Here's how the part is built. I have some questions about the finished solid (model axes, mm). Coordinates: 2 decimals unless noted, no trailing zeros. Write each loop counter-clockwise with the first axis right and the second up, starting at its lowest first coordinate (ties: lowest second). Pieces come first, ordered by that corner, then holes. Notation, with made-up numbers: (-18, 73.25) -> (1, 73.25) arc R19 cw to (1, 89.25) -> close; hole circle Ø8 at (-25, -38.75). An arc over 180 degrees is marked (long way). Use a Markdown table: item, result. Add a question column.
Item 1: If we mould it in two halves opening along Y, with no side actions, what happens to faces 1 (the cylindrical face through (-0.867, 3.905, 4.933)), 2 (the flat face through (2, 1, 10)), 3 (the cylindrical face through (1.438, -0.748, 4.933))? For each: pulls with the +Y half, pulls with the -Y half, needs draft (parallel to the pull), parting line crosses it, or undercut.
Item 2: If I drill on line 1 along Y through (x, z) = (0, 4.75); line 2 along X through (y, z) = (1, 4.5); line 3 along Y through (x, z) = (2.5, 3), over which ranges is the centre line in solid material (lowest first)? Write a range as from..to.
Item 3: Will these pins go through, and if not, where does the flat tip stop? pin 1 Ø1 at (y, z) = (1, 8.5) entering from -X; pin 2 Ø3.5 at (x, y) = (0, 0) entering from +Z.
Item 4: Imagine slicing it at A-A, the plane x = 0. Write out the boundary of the cut face in (y, z).
Item 5: Imagine slicing it at C-C, the plane z = 0.75. Write out the boundary of the cut face in (x, y), and give its area (3 significant figures).
Autodesk Inventor part; units mm, degrees
ref_plane "YZ Plane" through (0, 0, 0) normal (1, 0, 0) x (0, 1, 0)
ref_plane "XZ Plane" through (0, 0, 0) normal (0, 1, 0) x (-1, 0, 0)
ref_plane "XY Plane" through (0, 0, 0) normal (0, 0, 1) x (1, 0, 0)
sketch "スケッチ1" plane through (0, 0, 0) normal (0, 0, 1) x (1, 0, 0)
  circle A0 centre (0, 0) radius 4
  dimension "d13" = 8
extrude "押し出し1" add sketch "スケッチ1" along normal blind 10
sketch "スケッチ2" plane through (0, 0, 10) normal (0, 0, 1) x (1, 0, 0)
  point P0 (0, 0)
  point P1 (0, 0)
hole "穴1" at (0, 0, 10) direction (0, 0, -1) diameter 3.242 end through all
chamfer "面取り1" distance 0.2 angle 45 4 edges at (0, 1.621, 10) (0, 1.621, 0) (-4, 0, 10) (-4, 0, 0)
properties part number "ARF-410E" material "鋼、炭素鋼"
Ans:
| question | item | result |
|---|---|---|
| 1 | face 1 | parting line crosses it |
| 1 | face 2 | needs draft |
| 1 | face 3 | undercut |
| 2 | line 1 | y = -4..-1.62, 1.62..4 |
| 2 | line 2 | x = -3.87..-1.28, 1.28..3.87 |
| 2 | line 3 | y = -3.12..3.12 |
| 3 | pin 1 | stops at x = -3.97 |
| 3 | pin 2 | stops at z = 9.93 |
| 4 | outline | (-4, 0.2) -> (-3.8, 0) -> (-1.82, 0) -> (-1.62, 0.2) -> (-1.62, 9.8) -> (-1.82, 10) -> (-3.8, 10) -> (-4, 9.8) -> close; (1.62, 0.2) -> (1.82, 0) -> (3.8, 0) -> (4, 0.2) -> (4, 9.8) -> (3.8, 10) -> (1.82, 10) -> (1.62, 9.8) -> close |
| 5 | outline | circle Ø8 at (0, 0); hole circle Ø3.24 at (0, 0) |
| 5 | area | 42.0 mm^2 |
